Autodesk Inventor part; units mm, degrees
ref_plane "YZ Plane" through (0, 0, 0) normal (1, 0, 0) x (0, 1, 0)
ref_plane "XZ Plane" through (0, 0, 0) normal (0, 1, 0) x (-1, 0, 0)
ref_plane "XY Plane" through (0, 0, 0) normal (0, 0, 1) x (1, 0, 0)
sketch "Boceto1" plane through (0, 0, 0) normal (0, 0, 1) x (1, 0, 0)
  circle A0 centre (0, 0) radius 21.75
  arc A1 (1.304413, 21.71085) -> (0, 23.055) centre (0, 21.75) ccw
  arc A2 (0, 23.055) -> (-1.304413, 21.71085) centre (0, 21.75) ccw
  line L0 (0, -21.75) -> (0, -23.25)
  arc A3 (0, -23.25) -> (1.499108, -21.698276) centre (0, -21.75) ccw
  arc A4 (-1.499108, -21.698276) -> (0, -23.25) centre (0, -21.75) ccw
  line L1 (21.75, 0) -> (23.055, 0)
  line L2 (-21.75, 0) -> (-23.25, 0)
  arc A5 (-21.698276, 1.499108) -> (-21.698276, -1.499108) centre (-21.75, 0) ccw
  arc A6 (21.71085, -1.304413) -> (21.71085, 1.304413) centre (21.75, 0) ccw
  dimension "d0" = 43.5
  dimension "d2" = 1.5
  dimension "d4" = 1.5
extrude "Extrusión1" add sketch "Boceto1" along normal blind 81
sketch "Boceto2" plane through (0, 0, 81) normal (0, 0, 1) x (1, 0, 0)
  line L0 (0, 5) -> (4.330127, 2.5)
  line L1 (4.330127, 2.5) -> (4.330127, -2.5)
  line L2 (4.330127, -2.5) -> (0, -5)
  line L3 (0, -5) -> (-4.330127, -2.5)
  line L4 (-4.330127, -2.5) -> (-4.330127, 2.5)
  line L5 (-4.330127, 2.5) -> (0, 5)
  point P0 (0, 0)
  point P1 (0, 0)
extrude "Extrusión2" add sketch "Boceto2" along normal blind 20
sketch "Boceto10" plane through (0, 0, 0) normal (0, 0, -1) x (-1, 0, 0)
  circle A0 centre (0, 0) radius 7.5
  dimension "d37" = 15
extrude "Extrusión9" add sketch "Boceto10" along normal blind 30
sketch "Boceto12" plane through (0, 0, 0) normal (0, 0, -1) x (-1, 0, 0)
  circle A0 centre (0, 0) radius 10
  dimension "d40" = 20
extrude "Extrusión10" add sketch "Boceto12" along normal blind 30
sketch "Boceto20" plane through (0, 0, 81) normal (0, 0, 1) x (1, 0, 0)
  circle A0 centre (0, 0) radius 15
  dimension "d61" = 30
ref_plane "Plano de trabajo1" through (0, 0, 91) normal (0, 0, 1) x (1, 0, 0)
sketch "Boceto21" plane through (0, 0, 91) normal (0, 0, 1) x (1, 0, 0)
  line L0 (4.330127, 2.5) -> (4.330127, -2.5)
  circle A0 centre (0, 0) radius 5
sketch "Boceto20 outline for Solevación1" plane through (0, 0, 81) normal (0, 0, 1) x (1, 0, 0)
  circle A0 centre (0, 0) radius 15
sketch "Boceto21 outline for Solevación1" plane through (0, 0, 91) normal (0, 0, 1) x (1, 0, 0)
  circle A0 centre (0, 0) radius 5
loft "Solevación1" add profiles "Boceto20 outline for Solevación1", "Boceto21 outline for Solevación1"
sketch "Boceto22" plane through (0, 0, 81) normal (0, 0, 1) x (1, 0, 0)
  arc A0 (1.304413, 21.71085) -> (-1.304413, 21.71085) centre (0, 21.75) ccw
  arc A1 (1.304413, 21.71085) -> (-1.304413, 21.71085) centre (0, 21.749554) ccw
  arc A2 (21.71085, -1.304413) -> (21.71085, 1.304413) centre (21.75, 0) ccw
  arc A3 (21.71085, -1.304413) -> (21.71085, 1.304413) centre (21.749554, 0) ccw
  arc A4 (-1.499108, -21.698276) -> (1.499108, -21.698276) centre (0, -21.75) ccw
  arc A5 (-1.499108, -21.698276) -> (1.499108, -21.698276) centre (0, -21.749411) ccw
  arc A6 (-21.698276, 1.499108) -> (-21.698276, -1.499108) centre (-21.75, 0) ccw
  arc A7 (-21.685394, 1.49099) -> (-21.698276, -1.499108) centre (-21.753079, -0.003795) ccw
  arc A8 (-21.698276, 1.499108) -> (-21.698276, -1.499108) centre (-1.222086, 0) ccw
  arc A9 (1.304413, 21.71085) -> (-1.304413, 21.71085) centre (0, -0.250446) ccw
  arc A10 (21.71085, -1.304413) -> (21.71085, 1.304413) centre (-0.250446, 0) ccw
  arc A11 (-1.499108, -21.698276) -> (1.499108, -21.698276) centre (0, 0.250589) ccw
  point P0 (0, 0)
sketch "Boceto22 outline for Extrusión16" plane through (0, 0, 81) normal (0, 0, 1) x (1, 0, 0)
  arc A0 (-1.304413, 21.71085) -> (1.304413, 21.71085) centre (0, -0.250446) cw
  arc A1 (1.304413, 21.71085) -> (-1.304413, 21.71085) centre (0, 21.75) ccw
  arc A2 (21.71085, 1.304413) -> (21.71085, -1.304413) centre (-0.250446, 0) cw
  arc A3 (21.71085, -1.304413) -> (21.71085, 1.304413) centre (21.75, 0) ccw
  arc A4 (-21.698276, -1.499108) -> (-21.698276, 1.499108) centre (-1.222086, 0) cw
  arc A5 (-21.698276, 1.499108) -> (-21.698276, -1.499108) centre (-21.75, 0) ccw
  arc A6 (1.499108, -21.698276) -> (-1.499108, -21.698276) centre (0, 0.250589) cw
  arc A7 (-1.499108, -21.698276) -> (1.499108, -21.698276) centre (0, -21.75) ccw
extrude "Extrusión16" cut sketch "Boceto22 outline for Extrusión16" against normal blind 211
properties part number "eix bobina"
Check sheet for the modelled part. Datum: model origin and axes. Units: mm. A direction names the side the tool comes from. Round coordinates to 2 decimals unless told otherwise and drop trailing zeros. Loops run counter-clockwise (first coordinate to the right, second up) from the corner with the lowest first, then second, coordinate; pieces in that order, holes last. Notation, with made-up numbers: (-3.75, -11.75) -> (13.25, -11.75) arc R10 cw to (13.25, 2.25) -> close; hole circle Ø2 at (-37, -24.75). An arc over 180 degrees is marked (long way). Answer in a Markdown table with one row per item.
Q1. Set-up check for faces 1 (the face through (2.17, 9.76, -14.79)), 2 (the face through (-4.33, 0, 96)), 3 (the face through (4.33, 0, 96)), 4 (the face through (-2.3, -3.9, 91)): record each of +Z, -Z, +X, -X, +Y, -Y from which the full face is reachable in a straight line by a thin tool's end or side.
Data:
| item | result |
|---|---|
| face 1 | -Z |
| face 2 | +Z, -X, +Y, -Y |
| face 3 | +Z, +X, +Y, -Y |
| face 4 | +Z, -X, -Y |
Q2. Sectioned sample at B-B on x = 17. Enter the section's corners in (y, z).
Data:
| item | result |
|---|---|
| outline | (-13.57, 0) -> (13.57, 0) -> (13.57, 81) -> (-13.57, 81) -> close |
Q3. Sectioned sample at A-A on z = 33. Enter the section's corners in (x, y).
Data:
| item | result |
|---|---|
| outline | (-21.7, -1.5) arc R21.75 ccw to (-1.5, -21.7) arc R22 ccw to (1.5, -21.7) arc R21.75 ccw to (21.71, -1.3) arc R22 ccw to (21.71, 1.3) arc R21.75 ccw to (1.3, 21.71) arc R22 ccw to (-1.3, 21.71) arc R21.75 ccw to (-21.7, 1.5) arc R20.53 ccw to start |
Q4. Go/stop test with flat-tipped pins: P1, Ø1.5, axis at y = 1, z = 98, coming from the -X side; P2, Ø6, axis at y = -9, z = 57.5, coming from the -X side; P3, Ø5, axis at x = 8, y = 12, coming from the -Z side. Record where each tip stops, or that it passes through.
Data:
| item | result |
|---|---|
| P1 | stops at x = -4.33 |
| P2 | stops at x = -20.91 |
| P3 | stops at z = 0 |
Q5. Thickness scan on L1, parallel to Z at x = -16.5, y = -10; L2, parallel to Y at x = -1, z = 42. Record the ranges inside material, lowest first.
Data:
| item | result |
|---|---|
| L1 | z = 0 to 81 |
| L2 | y = -21.73 to 21.73 |
Q6. Release check for a two-part mould opening along Z. For faces 5 (the face through (-21.753, 0.021, 41.067)), 6 (the face through (5, 15, 81)), 7 (the face through (0, 0, -30)) record: released by +Z, released by -Z, zero draft, split by the parting line, or undercut.
Data:
| item | result |
|---|---|
| face 5 | zero draft |
| face 6 | released by +Z |
| face 7 | released by -Z |
Q7. Sectioned sample at C-C on z = -3.5. Enter the section's corners in (x, y), then the cut area to 3 significant figures.
Data:
| item | result |
|---|---|
| outline | circle Ø20 at (0, 0) |
| area | 314 mm^2 |
Q8. Sectioned sample at D-D on x = -16.5. Enter the section's corners in (y, z).
Data:
| item | result |
|---|---|
| outline | (-14.17, 0) -> (14.17, 0) -> (14.17, 81) -> (-14.17, 81) -> close |
